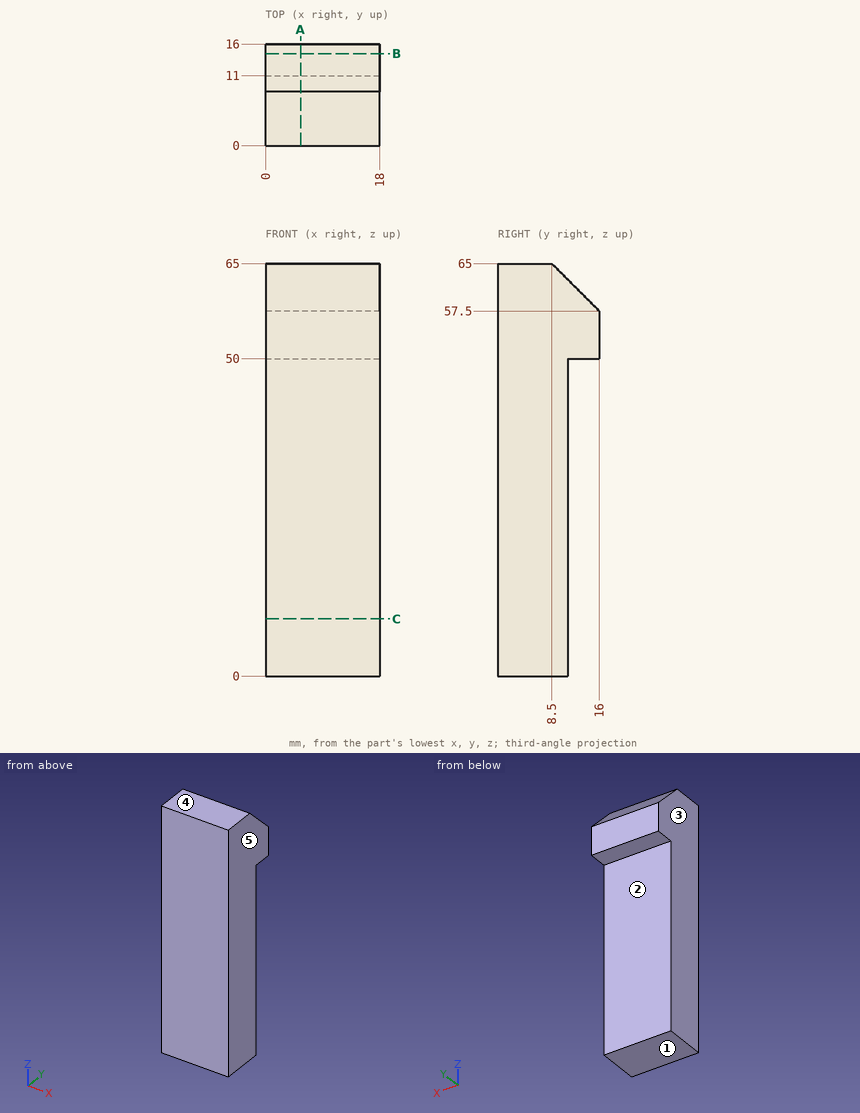
Here's the drawing with two shaded views (mm, measured from the low corner). I have some questions. A direction names the side the tool comes from. Coordinates: 2 decimals unless noted, no trailing zeros. Write each loop counter-clockwise with the first axis right and the second up, starting at its lowest first coordinate (ties: lowest second). Pieces come first, ordered by that corner, then holes.
Item 1: I want a section at C-C on z = 9. Write out the boundary of the cut face in (x, y), and give its area (3 significant figures).
Item 2: Will these pins go through, and if not, where does the flat tip stop? pin 1 (5 mm diameter, centred on x = 5.5, z = 35.5, fed in from -Y); pin 2 (4 mm diameter, centred on x = 7, y = 14.5, fed in from +Z); pin 3 (1.5 mm diameter, centred on x = 12, z = 37.5, fed in from +Y); pin 4 (3 mm diameter, centred on x = 4.5, y = 14, fed in from -Z).
Item 3: I want a section at B-B on y = 14.5. Write out the boundary of the cut face in (x, z), and give its area (3 significant figures).
Item 4: If we mould it in two halves opening along X, with no side actions, what happens to the marked faces 3, 4 and 5? For each: +X half, -X half, draft (parallel to the pull), parting line (faces both ways), or undercut.
Item 5: On a 3-axis mill with a long thin cutter (end or side, diameter ignored), from which of +Z, -Z, +X, -X, +Y, -Y can I reach the whole of each face in a straight line? I mean the marked faces 1 and 2. Say none if no direction works.
Item 6: I want a section at A-A on x = 5.5. Write out the boundary of the cut face in (y, z).
Item 7: If I drill on line 1 (Y direction, x = 5, z = 28); line 2 (Z direction, x = 16.25, y = 14); line 3 (Z direction, x = 1.25, y = 10.5), over which ranges is the centre line in solid material (lowest first)?
Findings below:
1. outline: (0, 0) - (18, 0) - (18, 11) - (0, 11) - close
1. area: 198 mm2
2. pin 1: stops at y = 0
2. pin 2: stops at z = 61
2. pin 3: stops at y = 11
2. pin 4: stops at z = 50
3. outline: (0, 50) - (18, 50) - (18, 59) - (0, 59) - close
3. area: 162 mm2
4. face 3: -X half
4. face 4: draft
4. face 5: +X half
5. face 1: -Z, +X, -X, +Y, -Y
5. face 2: -Z, +X, -X, +Y
6. outline: (0, 0) - (11, 0) - (11, 50) - (16, 50) - (16, 57.5) - (8.5, 65) - (0, 65) - close
7. line 1: y = 0 to 11
7. line 2: z = 50 to 59.5
7. line 3: z = 0 to 63
